The listing builds one solid part. Answer for the finished solid, in the listing's coordinates (mm). A direction names the side the tool comes from. Coordinates: 2 decimals unless noted, no trailing zeros. Write each loop counter-clockwise with the first axis right and the second up, starting at its lowest first coordinate (ties: lowest second). Pieces come first, ordered by that corner, then holes.
(1) The part is cut by section C-C on z = 4.25. Determine the outline of the cut face in (x, y).
(2) Straight lines are drawn through the part: line 1 (Y direction, x = -10.5, z = 17.4); line 2 (Z direction, x = -17, y = 11.75); line 3 (Y direction, x = 18, z = 9). For each, find the intervals that lie inside material, in ascending order.
(3) Given P1, Ø4, axis at x = -10.5, y = 7, coming from the -Z side; P2, Ø8, axis at x = -20, z = -8, coming from the -Y side; P3, Ø2, axis at x = -3.5, z = -5.5, coming from the -Y side; P4, Ø7, axis at x = 26.5, y = 8.5, coming from the -Z side, each flat-ended and moving along its own axis, determine where each tip first touches the part or whether it passes through.
(4) The part is cut by section B-B on z = 11.75. Determine the outline of the cut face in (x, y), plus the area to 3 significant figures.
(5) The part is cut by section D-D on y = 21. Determine the outline of the cut face in (x, z), plus the area to 3 significant figures.
(6) Which of the six approach directions +Z, -Z, +X, -X, +Y, -Y give full straight-line access (tool end or side, diameter ignored) to faces 1 (the flat face through (-24, 1, 10.087)), 2 (the flat face through (20, 10, 17)), 3 (the cylindrical face through (11.7, 6.1, 17.7))?
(7) The part is cut by section A-A on x = 10.5. Give the number of separate pieces and of enclosed holes in the cut face, plus the area to 3 significant figures.
(8) For a pull along X with two mould halves and no side action, classify faces 4 (the cylindrical face through (-4.886, 13.425, 17.736)), 5 (the flat face through (20, 11, -13)), 6 (the cylindrical face through (-18.43, 0.99, -18.15)), 7 (the flat face through (24, 13, -13.75)) as +X half, -X half, draft (parallel to the pull), parting line (faces both ways), or undercut.
from build123d import *

# Parameters (mm, degrees)
SKETCH_1_W               = 58
SKETCH_1_H               = 37.5
EXTRUDE_1_DEPTH          = 26.5
SKETCH_3_W               = 8.53894027
SKETCH_3_H               = 24.5
SKETCH_3_W_2             = 28.5
SKETCH_3_H_2             = 25.319580512
CUT_EXTRUDE_1_DEPTH      = 67.466626964
CUT_EXTRUDE_2_DEPTH      = 43.341616644
CUT_EXTRUDE_2_DEPTH_BACK = 26
SKETCH_4_W               = 1
SKETCH_4_H               = 2
SKETCH_4_R               = 4
SKETCH_5_W               = 38
SKETCH_5_H               = 24.5
CUT_EXTRUDE_3_DEPTH      = 26
SKETCH_6_R               = 1.5
CUT_EXTRUDE_4_DEPTH      = 43.341616644
SKETCH_7_R               = 2
SKETCH_7_R_2             = 1.5
CUT_EXTRUDE_5_DEPTH      = 51.985291997


with BuildPart() as part:
    # 草图1 → 凸台-拉伸1 (new body)
    with BuildSketch(Plane(origin=(0, 0, 0), x_dir=(1, 0, 0), z_dir=(0, 1, 0))):
        Rectangle(SKETCH_1_W, SKETCH_1_H)
    extrude(amount=EXTRUDE_1_DEPTH)

    # 草图3 → 切除-拉伸1 (cut, through all)
    with BuildSketch(Plane(origin=(29, 0, 0), x_dir=(0, 0, -1), z_dir=(1, 0, 0))):
        with Locations((18.019470135, 14.25)):
            Rectangle(SKETCH_3_W, SKETCH_3_H)
        with Locations((-2.5, 14.659790256)):
            Rectangle(SKETCH_3_W_2, SKETCH_3_H_2)
    extrude(amount=-CUT_EXTRUDE_1_DEPTH, mode=Mode.SUBTRACT)

    # 草图4 → 切除-拉伸2 (cut, two sides: drawn at the far end of the back side and taken through both)
    with BuildSketch(Plane(origin=(0, 2, 0), x_dir=(1, 0, 0), z_dir=(0, 1, 0)).offset(-CUT_EXTRUDE_2_DEPTH_BACK)):
        with BuildLine():
            Line((-29, 18.75), (-29, 13.75))
            Line((-29, 13.75), (-20, 13.75))
            Line((-20, 13.75), (-20, 11.75))
            Line((-20, 11.75), (-19, 11.75))
            Line((-19, 11.75), (-19, 16.75))
            ThreePointArc((-19, 16.75), (-18.414213562, 18.164213562), (-17, 18.75))
            Line((-17, 18.75), (-29, 18.75))
        make_face()
        with BuildLine():
            Line((29, 18.75), (17, 18.75))
            ThreePointArc((17, 18.75), (18.414213562, 18.164213562), (19, 16.75))
            Line((19, 16.75), (19, 11.75))
            Line((19, 11.75), (20, 11.75))
            Line((20, 11.75), (20, 13.75))
            Line((20, 13.75), (29, 13.75))
            Line((29, 13.75), (29, 18.75))
        make_face()
        with Locations((-19.5, 10.75)):
            Rectangle(SKETCH_4_W, SKETCH_4_H)
        with Locations((19.5, 10.75)):
            Rectangle(SKETCH_4_W, SKETCH_4_H)
        with BuildLine():
            Line((20, -21.492429243), (29, -21.492429243))
            Line((29, -21.492429243), (29, -8.086828318))
            ThreePointArc((29, -8.086828318), (28.414213562, -9.50104188), (27, -10.086828318))
            Line((27, -10.086828318), (20, -10.086828318))
            Line((20, -10.086828318), (20, -21.492429243))
        make_face()
        with BuildLine():
            Line((-20, -21.492429243), (-29, -21.492429243))
            Line((-29, -21.492429243), (-29, -8.086828318))
            ThreePointArc((-29, -8.086828318), (-28.414213562, -9.50104188), (-27, -10.086828318))
            Line((-27, -10.086828318), (-20, -10.086828318))
            Line((-20, -10.086828318), (-20, -21.492429243))
        make_face()
        with Locations(Location((-10.5, 5.75, 0), (0, 0, 90))):
            Circle(SKETCH_4_R)
        with Locations(Location((0, -4.75, 0), (0, 0, 90))):
            Circle(SKETCH_4_R)
        with Locations(Location((10.5, 5.75, 0), (0, 0, 90))):
            Circle(SKETCH_4_R)
    extrude(amount=CUT_EXTRUDE_2_DEPTH + CUT_EXTRUDE_2_DEPTH_BACK, mode=Mode.SUBTRACT)

    # 草图5 → 切除-拉伸3 (cut)
    with BuildSketch(Plane(origin=(0, 0, -13.75), x_dir=(-1, 0, 0), z_dir=(0, 0, -1))):
        with Locations((0, 14.25)):
            Rectangle(SKETCH_5_W, SKETCH_5_H)
    extrude(amount=-CUT_EXTRUDE_3_DEPTH, mode=Mode.SUBTRACT)

    # 草图6 → 切除-拉伸4 (cut, through all)
    with BuildSketch(Plane(origin=(0, 2, 0), x_dir=(1, 0, 0), z_dir=(0, 1, 0))):
        with Locations(Location((-26.5, 5.75, 0), (0, 0, 270))):
            Circle(SKETCH_6_R)
        with Locations(Location((-26.5, -4.25, 0), (0, 0, 270))):
            Circle(SKETCH_6_R)
        with Locations(Location((-17.5, 5.75, 0), (0, 0, 270))):
            Circle(SKETCH_6_R)
        with Locations(Location((-10.5, 12.75, 0), (0, 0, 270))):
            Circle(SKETCH_6_R)
        with Locations(Location((10.5, 12.75, 0), (0, 0, 270))):
            Circle(SKETCH_6_R)
        with Locations(Location((-3.5, 5.75, 0), (0, 0, 270))):
            Circle(SKETCH_6_R)
        with Locations(Location((0, 2.25, 0), (0, 0, 270))):
            Circle(SKETCH_6_R)
        with Locations(Location((3.5, 5.75, 0), (0, 0, 270))):
            Circle(SKETCH_6_R)
        with Locations(Location((-10.5, -1.25, 0), (0, 0, 270))):
            Circle(SKETCH_6_R)
        with Locations(Location((-7, -4.75, 0), (0, 0, 270))):
            Circle(SKETCH_6_R)
        with Locations(Location((0, -11.75, 0), (0, 0, 270))):
            Circle(SKETCH_6_R)
        with Locations(Location((7, -4.75, 0), (0, 0, 270))):
            Circle(SKETCH_6_R)
        with Locations(Location((10.5, -1.25, 0), (0, 0, 270))):
            Circle(SKETCH_6_R)
        with Locations(Location((17.5, 5.75, 0), (0, 0, 270))):
            Circle(SKETCH_6_R)
        with Locations(Location((26.5, 5.75, 0), (0, 0, 270))):
            Circle(SKETCH_6_R)
        with Locations(Location((26.5, -4.25, 0), (0, 0, 270))):
            Circle(SKETCH_6_R)
    extrude(amount=-CUT_EXTRUDE_4_DEPTH, mode=Mode.SUBTRACT)

    # 草图7 → 切除-拉伸5 (cut, through all)
    with BuildSketch(Plane(origin=(0, 0, -13.75), x_dir=(-1, 0, 0), z_dir=(0, 0, -1))):
        with BuildLine():
            ThreePointArc((-29, 22), (-27.681980515, 25.181980515), (-24.5, 26.5))
            Line((-24.5, 26.5), (-29, 26.5))
            Line((-29, 26.5), (-29, 22))
        make_face()
        with BuildLine():
            ThreePointArc((-24.5, 26.5), (-21.318019485, 25.181980515), (-20, 22))
            Line((-20, 22), (-20, 24.5))
            Line((-20, 24.5), (-20, 26.5))
            Line((-20, 26.5), (-24.5, 26.5))
        make_face()
        with Locations((-24.502255963, 20)):
            Circle(SKETCH_7_R)
        with Locations((-24.502255963, 8)):
            Circle(SKETCH_7_R)
        with BuildLine():
            Line((-20, 26.5), (-20, 24.5))
            ThreePointArc((-20, 24.5), (-19.414213562, 25.914213562), (-18, 26.5))
            Line((-18, 26.5), (-20, 26.5))
        make_face()
        with BuildLine():
            Line((24.502255963, 26.5), (18, 26.5))
            ThreePointArc((18, 26.5), (19.414213562, 25.914213562), (20, 24.5))
            Line((20, 24.5), (20.002255963, 22))
            ThreePointArc((20.002255963, 22), (21.320275448, 25.181980515), (24.502255963, 26.5))
        make_face()
        with BuildLine():
            Line((29, 26.5), (24.502255963, 26.5))
            ThreePointArc((24.502255963, 26.5), (27.684236479, 25.181980515), (29.002255963, 22))
            Line((29.002255963, 22), (29, 26.5))
        make_face()
        with Locations((24.502255963, 20)):
            Circle(SKETCH_7_R)
        with Locations((10.5, 21)):
            Circle(SKETCH_7_R_2)
        with Locations((-10.5, 7)):
            Circle(SKETCH_7_R_2)
        with Locations((3.5, 14)):
            Circle(SKETCH_7_R_2)
        with Locations((10.5, 14)):
            Circle(SKETCH_7_R_2)
        with Locations((17.5, 14)):
            Circle(SKETCH_7_R_2)
        with Locations((24.502255963, 8)):
            Circle(SKETCH_7_R)
        with Locations((10.5, 7)):
            Circle(SKETCH_7_R_2)
        with Locations((-17.5, 14)):
            Circle(SKETCH_7_R_2)
        with Locations((-10.5, 14)):
            Circle(SKETCH_7_R_2)
        with Locations((-10.5, 21)):
            Circle(SKETCH_7_R_2)
        with Locations((-3.5, 14)):
            Circle(SKETCH_7_R_2)
    extrude(amount=-CUT_EXTRUDE_5_DEPTH, mode=Mode.SUBTRACT)


solid = part.part
Model answer:
1. outline: (-29, 0) - (-28, 0) - (-28, 2) - (-29, 2) - close; (-25, 0) - (-8.41, 0) - (-8.41, 2) - (-25, 2) - close; (-5.59, 0) - (-3.97, 0) - (-3.97, 2) - (-5.59, 2) - close; (3.97, 0) - (5.59, 0) - (5.59, 2) - (3.97, 2) - close; (8.41, 0) - (25, 0) - (25, 2) - (8.41, 2) - close; (28, 0) - (29, 0) - (29, 2) - (28, 2) - close
2. line 1: y = 0 to 5.5, 8.5 to 12.5, 15.5 to 19.5, 22.5 to 26.5
2. line 2: z = 16.75 to 18.75
2. line 3: y = 0 to 2
3. P1: stops at z = 16.75
3. P2: stops at y = 0
3. P3: passes through
3. P4: stops at z = -13.75
4. outline: (-20, 0) - (-1.5, 0) - (-1.5, 2) - (-20, 2) - close; (1.5, 0) - (20, 0) - (20, 2) - (1.5, 2) - close
4. area: 74.0 mm2
5. outline: (-29, -13.75) - (-26.23, -13.75) - (-26.23, -11.75) - (-29, -11.75) - close; (-22.77, -13.75) - (-20, -13.75) - (-20, -11.75) - (-22.77, -11.75) - close; (-20, 16.75) - (-12, 16.75) - (-12, 18.75) - (-20, 18.75) - close; (-9, 16.75) - (9, 16.75) - (9, 18.75) - (-9, 18.75) - close; (12, 16.75) - (20, 16.75) - (20, 18.75) - (12, 18.75) - close; (20, -13.75) - (22.77, -13.75) - (22.77, -11.75) - (20, -11.75) - close; (26.23, -13.75) - (29, -13.75) - (29, -11.75) - (26.23, -11.75) - close
5. area: 90.1 mm2
6. face 1: +Z, -X, +Y, -Y
6. face 2: +Z, +X, +Y, -Y
6. face 3: +Z, -Z
7. separate pieces: 7
7. enclosed holes: 0
7. area: 78.0 mm2
8. face 4: undercut
8. face 5: undercut
8. face 6: -X half
8. face 7: draft
